```python
from build123d import *

# Parameters (mm, degrees)
F1_DEPTH = 47.0916
F0_R     = 10.16
F2_DEPTH = 25.4
F3_R     = 3.302


with BuildPart() as f1:
    # F0 (on Top) → F1 (new body)
    with BuildSketch(Plane.XY):
        with BuildLine():
            ThreePointArc((-42.087322, -25.984875), (-29.931071, -15.440859), (-25.4, 0))
            ThreePointArc((-25.4, 0), (-29.45069, 14.665908), (-40.454339, 25.173842))
            ThreePointArc((-40.454339, 25.173842), (-82.535454, 0.911648), (-42.087322, -25.984875))
        make_face()
        with BuildLine():
            ThreePointArc((-42.087322, -7.92564), (-68.142943, 1.844467), (-40.454339, 4.617833))
            Line((-40.454339, 4.617833), (-35.4457, 4.617833))
            Line((-35.4457, 4.617833), (-35.4457, -7.92564))
            Line((-35.4457, -7.92564), (-42.087322, -7.92564))
        make_face(mode=Mode.SUBTRACT)
    extrude(amount=F1_DEPTH)

    # F0 (on Top) → F2 (join)
    with BuildSketch(Plane.XY):
        with BuildLine():
            ThreePointArc((-40.454339, 25.173842), (-29.45069, 14.665908), (-25.4, 0))
            ThreePointArc((-25.4, 0), (-29.931071, -15.440859), (-42.087322, -25.984875))
            Line((-42.087322, -25.984875), (0, -19.069276))
            ThreePointArc((0, -19.069276), (15.96121, -0.271354), (0, 18.526568))
            Line((0, 18.526568), (-40.454339, 25.173842))
        make_face()
        Circle(F0_R, mode=Mode.SUBTRACT)
    extrude(amount=F2_DEPTH)

    # F3
    f3_edges = [f1.edges().sort_by_distance(p)[0] for p in [
        (-65.862678, 25.984875, 47.0916),
    ]]
    fillet(f3_edges, radius=F3_R)


solid = f1.part
```
Input: part model. Units: mm. Frame: model coordinates. A direction names the side the tool comes from. Coordinates: 2 decimals unless noted, no trailing zeros. Loops run counter-clockwise (first coordinate to the right, second up) from the corner with the lowest first, then second, coordinate; pieces in that order, holes last. Notation, with made-up numbers: (1.5, 2.5) - (36.5, 2.5) arc R30 cw to (36.5, 36.5) - close; hole circle Ø11 at (-38, -34). An arc over 180 degrees is marked (long way). Answer in a Markdown table with one row per item.
(1) Cut plane D-D on x = -13.5. Output: boundary loops of the cut face in (y, z).
Model answer:
| item | result |
|---|---|
| outline | (-21.29, 0) - (20.74, 0) - (20.74, 25.4) - (-21.29, 25.4) - close |
(2) Pin query (flat end, axial travel): P1, Ø1.5, axis at x = -38, z = 13.5, coming from the -Y side; P2, Ø15.5, axis at x = -18.5, y = -8, coming from the +Z side; P3, Ø6, axis at x = -0.5, z = 22, coming from the +Y side. Return the tip coordinate at first contact, or that it passes through.
Model answer:
| item | result |
|---|---|
| P1 | stops at y = -25.44 |
| P2 | stops at z = 25.4 |
| P3 | stops at y = 19.1 |
(3) Cut plane A-A on z = 12.5. Count the separate pieces of the cut face and the enclosed holes in it, plus the area to 3 significant figures.
Model answer:
| item | result |
|---|---|
| separate pieces | 1 |
| enclosed holes | 2 |
| area | 3,240 mm² |
(4) Set-up query: faces 1 (the face through (-19.944, 21.804, 12.522)), 2 (the face through (-39, -7.926, 23)). Return all of +Z, -Z, +X, -X, +Y, -Y with unobstructed straight access to the full face (end or side cutting, diameter ignored); none if empty.
Model answer:
| item | result |
|---|---|
| face 1 | +Z, -Z, +X, +Y |
| face 2 | +Z, -Z |
(5) Material intervals for L1, parallel to Y at x = -54, z = 38.5; L2, parallel to X at y = -6, z = 12.5; L3, parallel to X at y = 3.5, z = 15, sorted ascending. Write a range as from..to.
Model answer:
| item | result |
|---|---|
| L1 | y = -28.57..-14.29, 14.29..28.57 |
| L2 | x = -81.91..-66.94, -35.45..-8.2, 8.2..15.08 |
| L3 | x = -82.33..-67.83, -35.45..-9.54, 9.54..15.58 |
(6) Cut plane B-B on x = 2. Output: boundary loops of the cut face in (y, z).
Model answer:
| item | result |
|---|---|
| outline | (-18.63, 0) - (-9.96, 0) - (-9.96, 25.4) - (-18.63, 25.4) - close; (9.96, 0) - (18.09, 0) - (18.09, 25.4) - (9.96, 25.4) - close |
(7) Mould query, pull axis Y, two halves, no side actions, for faces 3 (the face through (-1.323, 10.074, 12.522)), 4 (the face through (-21.338, -22.575, 12.522)), 5 (the face through (-43, -11, 47.092)), 6 (the face through (-35.446, -2, 23)). Classes: pulls with the +Y half, pulls with the -Y half, needs draft (parallel to the pull), parting line crosses it, or undercut.
Model answer:
| item | result |
|---|---|
| face 3 | undercut |
| face 4 | pulls with the -Y half |
| face 5 | needs draft |
| face 6 | undercut |
